```python
from build123d import *

# Parameters (mm, degrees)
F1_DEPTH = 2
F2_W     = 2
F2_H     = 3
F3_DEPTH = 10
F4_R     = 0.99999


# Not quite as in the source:
# - a fillet or chamfer is up to 0.001 mm smaller than in the source, because OpenCascade refuses the exact size


with BuildPart() as f1:
    # F0 (on Top) → F1 (new body)
    with BuildSketch(Plane.XY):
        with BuildLine():
            Line((8.5, -100), (8.5, 0))
            ThreePointArc((8.5, 0), (0, 8.5), (-8.5, 0))
            Line((-8.5, 0), (-8.5, -100))
            ThreePointArc((-8.5, -100), (0, -108.5), (8.5, -100))
        make_face()
        with BuildLine():
            ThreePointArc((-2, 4.582575695), (0, 5), (2, 4.582575695))
            Line((2, 4.582575695), (2, -4.582575695))
            ThreePointArc((2, -4.582575695), (0, -5), (-2, -4.582575695))
            Line((-2, -4.582575695), (-2, 4.582575695))
        make_face(mode=Mode.SUBTRACT)
    extrude(amount=F1_DEPTH)

    # F2 (on Top) → F3 (join)
    with BuildSketch(Plane.XY):
        with Locations((-9.5, -1.5)):
            Rectangle(F2_W, F2_H)
        with BuildLine():
            Line((0, 10.5), (0, 8.5))
            ThreePointArc((0, 8.5), (1.5247314005, 8.3621285661), (3, 7.9529868603))
            Line((3, 7.9529868603), (3, 10.5))
            Line((3, 10.5), (0, 10.5))
        make_face()
    extrude(amount=F3_DEPTH)

    # F4 (radius 1 in the source; OpenCascade refuses exactly that, so slightly less here)
    f4_edges = [f1.edges().sort_by_distance(p)[0] for p in [
        (-8.5, 0, 1),
        (0, 8.5, 1),
        (-8.5, -3, 1),
        (-10.5, -1.5, 0),
        (1.5, 10.5, 0),
        (3, 7.952987, 1),
    ]]
    fillet(f4_edges, radius=F4_R)


solid = f1.part
```
Model file for the job. Use its own axes, mm. A direction names the side the tool comes from. Give positions to 0.01 mm unless a question says otherwise; leave off trailing zeros. Loops run counter-clockwise (first coordinate to the right, second up) from the corner with the lowest first, then second, coordinate; pieces in that order, holes last. Notation, with made-up numbers: (-28.75, 1) -> (25.25, 1) arc R18 cw to (25.25, 12) -> close; hole circle Ø1 at (58, 2). An arc over 180 degrees is marked (long way). Use CSV: the item, a comma, the result in double quotes. Start each with the question number.
1) Flat gauge pins, fed straight in: pin 1 Ø0.6 at (y, z) = (-47.5, 0.5) entering from -X; pin 2 Ø6 at (x, y) = (-2, -63) entering from +Z; pin 3 Ø3 at (y, z) = (9.5, 3.5) entering from +X. Where does each tip first touch, or does it go through?
2) Mould opens along Y. For faces 1 (the flat face through (-1, -49, 2)), 2 (the cylindrical face through (0, -5, 1)), 3 (the flat face through (-2, 0, 1)), 4 (the flat face through (-10, -3, 5)) say: released by +Y, released by -Y, zero draft, split by the parting line, or undercut.
3) Tool access for faces 5 (the flat face through (3, 9, 5)), 6 (the cylindrical face through (1.504, 8.366, 5.944)), 7 (the flat face through (-10, 0, 5)): list every direction of +Z, -Z, +X, -X, +Y, -Y with a clear straight run to the whole face (end or side of a thin tool).
4) Slice it at A-A on z = 6. Give the cut face in (x, y).
5) Wall check: line 1 (Z direction, x = -0.5, y = -40); line 2 (X direction, y = 1.5, z = 1.5); line 3 (X direction, y = -35, z = 1.5). Give the ranges that are in metal, low to high.
6) Slice it at B-B on y = -31.5. Give the cut face in (x, z), plus the area to 3 significant figures.
7) Slice it at C-C on x = 6.5. Give the cut face in (y, z), plus the area to 3 significant figures.
Computed values:
1,pin 1,"stops at x = -8.5"
1,pin 2,"stops at z = 2"
1,pin 3,"stops at x = 3"
2,face 1,"zero draft"
2,face 2,"undercut"
2,face 3,"undercut"
2,face 4,"released by -Y"
3,face 5,"+Z, +X, +Y"
3,face 6,"+Z, -X, -Y"
3,face 7,"+Z, -X, +Y"
4,outline,"(-10.5, -3) -> (-8.5, -3) -> (-8.5, 0) -> (-10.5, 0) -> close; (0, 8.5) arc R8.5 cw to (3, 7.95) -> (3, 10.5) -> (0, 10.5) -> close"
5,line 1,"z = 0 to 2"
5,line 2,"x = -8.37 to -2, 2 to 8.37"
5,line 3,"x = -8.5 to 8.5"
6,outline,"(-8.5, 0) -> (8.5, 0) -> (8.5, 2) -> (-8.5, 2) -> close"
6,area,"34.0 mm^2"
7,outline,"(-105.48, 0) -> (5.48, 0) -> (5.48, 2) -> (-105.48, 2) -> close"
7,area,"222 mm^2"
